Autodesk Inventor part; units mm, degrees
ref_plane "YZ Plane" through (0, 0, 0) normal (1, 0, 0) x (0, 1, 0)
ref_plane "XZ Plane" through (0, 0, 0) normal (0, 1, 0) x (-1, 0, 0)
ref_plane "XY Plane" through (0, 0, 0) normal (0, 0, 1) x (1, 0, 0)
sketch "草圖1" plane through (0, 0, 0) normal (0, 1, 0) x (-1, 0, 0)
  line L0 (0, 0) -> (30, 0)
  line L1 (30, 0) -> (30, -100)
  line L2 (30, -100) -> (0, -100)
  line L3 (0, -100) -> (0, 0)
  dimension "d0" = 30
  dimension "d1" = 100
extrude "擠出1" add sketch "草圖1" along normal blind 50
sketch "草圖2" plane through (0, 50, 0) normal (0, 1, 0) x (1, 0, 0)
  line L0 (-11.3304, 13.4262) -> (-3.3304, 13.4262)
  line L1 (-3.3304, 13.4262) -> (-3.3304, 5.4262)
  line L2 (-3.3304, 5.4262) -> (-11.3304, 5.4262)
  line L3 (-11.3304, 5.4262) -> (-11.3304, 13.4262)
  point P0 (0, 0)
  dimension "d4" = 8
  dimension "d5" = 8
extrude "擠出2" cut sketch "草圖2" against normal blind 50
pattern_linear "矩形陣列1" count 9 spacing 10 along (0, 0, -1) of "擠出2"
pattern_linear "矩形陣列2" count 2 spacing 15 along (-1, 0, 0) of "擠出2", "矩形陣列1"
properties part number "矩形陣列"
CAD build for the part. Positions are in the model's coordinates, mm. A direction names the side the tool comes from. Round coordinates to 2 decimals unless told otherwise and drop trailing zeros. Loops run counter-clockwise (first coordinate to the right, second up) from the corner with the lowest first, then second, coordinate; pieces in that order, holes last.
(1) Which spindle directions (+Z, -Z, +X, -X, +Y, -Y) get a long thin tool onto all of the face, cutting with end or side? Do faces 1 (the flat face through (-15, 25, -100)), 2 (the flat face through (-26.33, 25, -49)). Say none if no direction does.
(2) Cut at B-B (x = -25). State how many separate pieces and enclosed holes the cut face has, plus the area to 3 significant figures.
(3) Cut at A-A (z = -37). Give the cut face in (x, y).
(4) Wall check: line 1 along X through (y, z) = (11, -41.5). Give the ranges that are in metal, low to high.
(5) Two-plate mould, pull along X, no slides. Class faces 3 (the flat face through (-22, 25, -33.426)), 4 (the flat face through (-15, 0, -49)): +X half, -X half, draft (parallel to the pull), parting line (faces both ways), or undercut.
Findings below:
1. face 1: -Z, +X, -X, +Y, -Y
1. face 2: +Y, -Y
2. separate pieces: 10
2. enclosed holes: 0
2. area: 1,400 mm2
3. outline: (-30, 0) - (-26.33, 0) - (-26.33, 50) - (-30, 50) - close; (-18.33, 0) - (-11.33, 0) - (-11.33, 50) - (-18.33, 50) - close; (-3.33, 0) - (0, 0) - (0, 50) - (-3.33, 50) - close
4. line 1: x = -30 to -26.33, -18.33 to -11.33, -3.33 to 0
5. face 3: undercut
5. face 4: draft
